Source: three-view drawing plus pictorial views. Frame: mm from the lowest corner of the part. Coordinates: 2 decimals unless noted, no trailing zeros. Order: outer loops, then holes, each group sorted by start corner. A loop starts at its lowest first (then second) coordinate and runs counter-clockwise, first axis right, second up. Notation, with made-up numbers: (89.5, -33.75) - (98.5, -33.75) arc R19 ccw to (98.5, -27.75) - close; hole circle Ø6 at (51.25, 88.25). An arc over 180 degrees is marked (long way). Use a Markdown table: item, result. Add a question column.
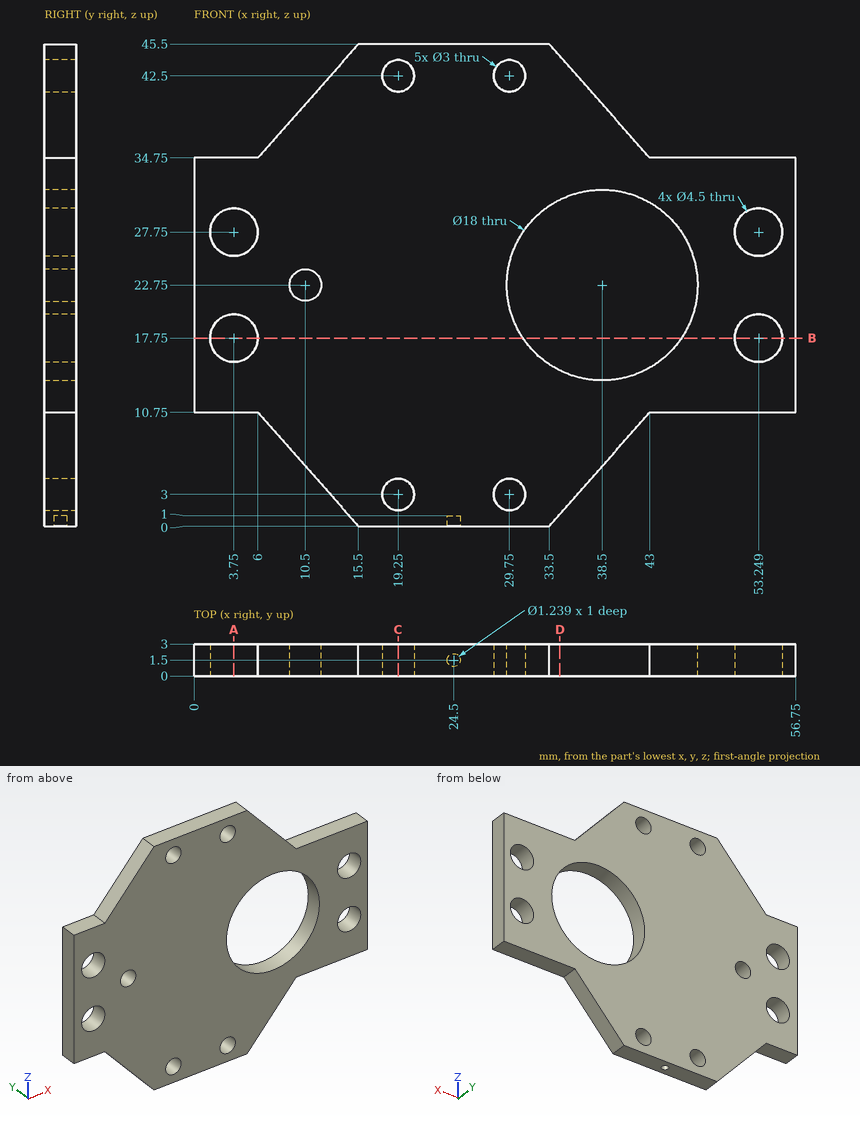
1) Section A-A (x = 3.75). Return loops of the section in (y, z).
2) Section D-D (x = 34.5). Return loops of the section in (y, z).
3) Ray query, line 1 along Z through (x, y) = (3.75, 0.8); line 2 along Z through (x, y) = (42, 2.9); line 3 along Z through (x, y) = (42.5, 2.5) (1 decimal). Return the intervals inside material, ascending.
4) Section B-B (z = 17.75). Return loops of the section in (x, y).
5) Pin query (flat end, axial travel): pin 1 (0.9 mm diameter, centred on x = 3.5, y = 2, fed in from +Z). Return the tip coordinate at first contact, or that it passes through.
6) Section C-C (x = 19.25). Return loops of the section in (y, z).
Values follow:
| question | item | result |
|---|---|---|
| 1 | outline | (0, 10.75) - (3, 10.75) - (3, 15.5) - (0, 15.5) - close; (0, 20) - (3, 20) - (3, 25.5) - (0, 25.5) - close; (0, 30) - (3, 30) - (3, 34.75) - (0, 34.75) - close |
| 2 | outline | (0, 1.13) - (3, 1.13) - (3, 14.69) - (0, 14.69) - close; (0, 30.81) - (3, 30.81) - (3, 44.37) - (0, 44.37) - close |
| 3 | line 1 | z = 10.75 to 15.5, 20 to 25.5, 30 to 34.75 |
| 3 | line 2 | z = 9.62 to 14.46, 31.04 to 35.88 |
| 3 | line 3 | z = 10.2 to 14.7, 30.8 to 35.3 |
| 4 | outline | (0, 0) - (1.5, 0) - (1.5, 3) - (0, 3) - close; (6, 0) - (31.02, 0) - (31.02, 3) - (6, 3) - close; (45.98, 0) - (51, 0) - (51, 3) - (45.98, 3) - close; (55.5, 0) - (56.75, 0) - (56.75, 3) - (55.5, 3) - close |
| 5 | pin 1 | stops at z = 34.75 |
| 6 | outline | (0, 0) - (3, 0) - (3, 1.5) - (0, 1.5) - close; (0, 4.5) - (3, 4.5) - (3, 41) - (0, 41) - close; (0, 44) - (3, 44) - (3, 45.5) - (0, 45.5) - close |
